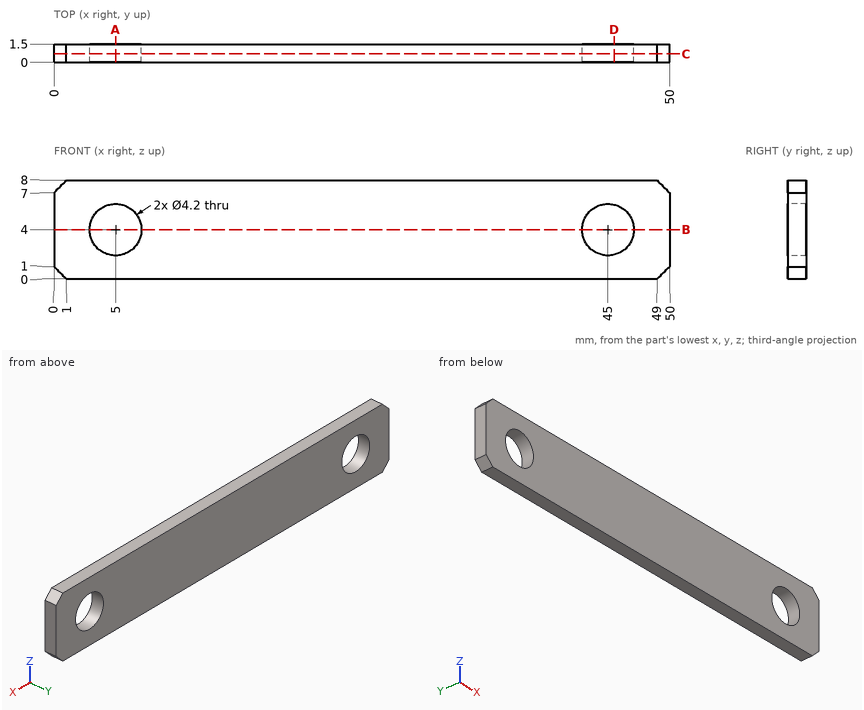
Check sheet for the drawn part. Datum: minimum x, y, z corner. Units: mm. Round coordinates to 2 decimals unless told otherwise and drop trailing zeros. Order: outer loops, then holes, each group sorted by start corner. A loop starts at its lowest first (then second) coordinate and runs counter-clockwise, first axis right, second up.
(1) Cross-section at D-D, the plane x = 45.5. Enter the section's corners in (y, z).
(2) Scan lines: probe 1 along X at (y, z) = (0.9, 4); probe 2 along Z at (x, y) = (45, 0.75); probe 3 along X at (y, z) = (0.35, 3.5). Record each from-to range of solid material in increasing order.
(3) Cross-section at A-A, the plane x = 5. Enter the section's corners in (y, z), and give its area (3 significant figures).
(4) Cross-section at C-C, the plane y = 0.7. Enter the section's corners in (x, z), and give its area (3 significant figures).
(5) Cross-section at B-B, the plane z = 4. Enter the section's corners in (x, y), and give its area (3 significant figures).
Check sheet entries:
1. outline: (0, 0) - (1.5, 0) - (1.5, 1.96) - (0, 1.96) - close; (0, 6.04) - (1.5, 6.04) - (1.5, 8) - (0, 8) - close
2. probe 1: x = 0 to 2.9, 7.1 to 42.9, 47.1 to 50
2. probe 2: z = 0 to 1.9, 6.1 to 8
2. probe 3: x = 0 to 2.96, 7.04 to 42.96, 47.04 to 50
3. outline: (0, 0) - (1.5, 0) - (1.5, 1.9) - (0, 1.9) - close; (0, 6.1) - (1.5, 6.1) - (1.5, 8) - (0, 8) - close
3. area: 5.70 mm2
4. outline: (0, 1) - (1, 0) - (49, 0) - (50, 1) - (50, 7) - (49, 8) - (1, 8) - (0, 7) - close; hole circle Ø4.2 at (5, 4); hole circle Ø4.2 at (45, 4)
4. area: 370 mm2
5. outline: (0, 0) - (2.9, 0) - (2.9, 1.5) - (0, 1.5) - close; (7.1, 0) - (42.9, 0) - (42.9, 1.5) - (7.1, 1.5) - close; (47.1, 0) - (50, 0) - (50, 1.5) - (47.1, 1.5) - close
5. area: 62.4 mm2
